For this review, take the finished solid that the model builds, in its own axes (mm). A direction names the side the tool comes from. Round coordinates to 2 decimals unless told otherwise and drop trailing zeros. Order: outer loops, then holes, each group sorted by start corner. A loop starts at its lowest first (then second) coordinate and runs counter-clockwise, first axis right, second up. Notation, with made-up numbers: (84, 74) - (103, 74) arc R17 cw to (103, 78) - close; hole circle Ø1 at (22, 31). An arc over 180 degrees is marked (long way). One line per item, written item: value.
Autodesk Inventor part; units mm, degrees
ref_plane "YZ Plane" through (0, 0, 0) normal (1, 0, 0) x (0, 1, 0)
ref_plane "XZ Plane" through (0, 0, 0) normal (0, 1, 0) x (-1, 0, 0)
ref_plane "XY Plane" through (0, 0, 0) normal (0, 0, 1) x (1, 0, 0)
sketch "Sketch2" plane through (0, 0, 0) normal (0, 1, 0) x (-1, 0, 0)
  line L0 (-9.525, 50.8) -> (9.525, 50.8)
  line L1 (9.525, 50.8) -> (9.525, -50.8)
  line L2 (9.525, -50.8) -> (-9.525, -50.8)
  line L3 (-9.525, -50.8) -> (-9.525, 50.8)
  line L4 (-9.525, 50.8) -> (9.525, -50.8) construction
  line L5 (9.525, 50.8) -> (-9.525, -50.8) construction
  line L6 (-9.525, 50.8) -> (5.715, 50.8)
  line L7 (5.715, 50.8) -> (5.715, 43.18)
  circle A0 centre (5.715, 43.18) radius 2.54
  line L8 (-9.525, -50.8) -> (5.715, -50.8)
  line L9 (5.715, -50.8) -> (5.715, -43.18)
  circle A1 centre (5.715, -43.18) radius 2.54
  point P0 (0, 0)
  dimension "d0" = 19.05
  dimension "d1" = 101.6
  dimension "d2" = 15.24
  dimension "d3" = 7.62
  dimension "d4" = 5.08
  dimension "d10" = 15.24
  dimension "d11" = 7.62
  dimension "d12" = 5.08
extrude "Extrusion3" add sketch "Sketch2" along normal blind 2.54
sketch "Sketch4" plane through (0, 2.54, 0) normal (0, 1, 0) x (1, 0, 0)
  line L0 (9.525, -50.8) -> (9.525, 50.8)
  line L1 (9.525, -50.8) -> (6.985, -50.8)
  line L2 (6.985, -50.8) -> (6.985, 50.8)
  line L3 (6.985, 50.8) -> (9.525, 50.8)
  line L4 (9.525, 50.8) -> (9.525, -50.8)
  point P0 (0, 0)
  dimension "d15" = 2.54
  dimension "d16" = 101.6
extrude "Extrusion4" add sketch "Sketch4" along normal blind 29.21
sketch "Sketch5" plane through (9.525, 0, 50.8) normal (1, 0, 0) x (0, 0, -1)
  line L0 (0, 0) -> (101.6, 0)
  line L1 (101.6, 0) -> (101.6, 31.75)
  line L2 (0, 31.75) -> (101.6, 31.75)
  line L3 (0, 0) -> (0, 31.75)
  line L4 (0, 31.75) -> (101.6, 31.75)
  line L5 (0, 31.75) -> (33.8658, 31.75)
  line L6 (33.8658, 31.75) -> (67.724, 31.75)
  line L7 (16.9329, 31.75) -> (16.9329, 19.05)
  line L8 (50.7949, 31.75) -> (50.7949, 19.05)
  line L9 (67.724, 31.75) -> (101.6, 31.75)
  line L10 (84.662, 31.75) -> (84.662, 19.05)
  line L11 (16.9329, 19.05) -> (4.6829, 19.05)
  line L12 (4.6829, 19.05) -> (29.1829, 19.05)
  line L13 (50.7949, 19.05) -> (38.5449, 19.05)
  line L14 (38.5449, 19.05) -> (63.0449, 19.05)
  circle A0 centre (4.6829, 19.05) radius 1.651
  circle A1 centre (29.1829, 19.05) radius 1.651
  circle A2 centre (38.5449, 19.05) radius 1.651
  circle A3 centre (63.0449, 19.05) radius 1.651
  line L15 (7.4329, 13.55) -> (26.4329, 13.55)
  line L16 (26.4329, 13.55) -> (26.4329, 24.55)
  line L17 (26.4329, 24.55) -> (7.4329, 24.55)
  line L18 (7.4329, 24.55) -> (7.4329, 13.55)
  line L19 (7.4329, 13.55) -> (26.4329, 24.55) construction
  line L20 (26.4329, 13.55) -> (7.4329, 24.55) construction
  line L21 (41.2949, 13.55) -> (60.2949, 13.55)
  line L22 (60.2949, 13.55) -> (60.2949, 24.55)
  line L23 (60.2949, 24.55) -> (41.2949, 24.55)
  line L24 (41.2949, 24.55) -> (41.2949, 13.55)
  line L25 (41.2949, 13.55) -> (60.2949, 24.55) construction
  line L26 (60.2949, 13.55) -> (41.2949, 24.55) construction
  circle A4 centre (84.662, 19.05) radius 3.302
  point P0 (50.8, 0)
  dimension "d19" = 33.8658
  dimension "d20" = 33.8582
  dimension "d21" = 12.7
  dimension "d22" = 12.7
  dimension "d23" = 12.7
  dimension "d24" = 12.25
  dimension "d25" = 24.5
  dimension "d26" = 12.25
  dimension "d27" = 24.5
  dimension "d28" = 3.302
  dimension "d29" = 3.302
  dimension "d30" = 3.302
  dimension "d31" = 3.302
  dimension "d32" = 19
  dimension "d33" = 11
  dimension "d34" = 19
  dimension "d35" = 11
  dimension "d36" = 6.604
extrude "Extrusion5" cut sketch "Sketch5" against normal through all contours A4 | A3 | A2 | L23 L22 L14 L8 | L8 L13 L24 L23 | A0 | L17 L16 L12 L7 | L7 L11 L18 L17 | L12 L16 L15 L18 L11 | L14 L22 L21 L24 L13
properties part number "Pi-Output-Holder"
Item 1: Wall thickness on line 1 (Y direction, x = -3, z = 44); line 2 (X direction, y = 23.5, z = 18) (3 decimals); line 3 (Z direction, x = 8.5, y = 16): over which ranges is each line inside the solid? List them lowest first.
Returned:
line 1: 0 to 2.54
line 2: 6.985 to 9.525
line 3: -50.8 to -35.13, -32.6 to -9.49, 9.51 to 24.37, 43.37 to 50.8
Item 2: Take a section at C-C (z = -43.18). Write out the cut boundary in (x, y) (3 decimals), plus the area to 3 significant figures.
Returned:
outline: (-9.525, 0) - (-8.255, 0) - (-8.255, 2.54) - (-9.525, 2.54) - close; (-3.175, 0) - (9.525, 0) - (9.525, 31.75) - (6.985, 31.75) - (6.985, 2.54) - (-3.175, 2.54) - close
area: 110 mm^2
Item 3: Take a section at A-A (y = 19.05). Write out the cut boundary in (x, z) (3 decimals), plus the area to 3 significant figures.
Returned:
outline: (6.985, -50.8) - (9.525, -50.8) - (9.525, -37.164) - (6.985, -37.164) - close; (6.985, -30.56) - (9.525, -30.56) - (9.525, -13.896) - (6.985, -13.896) - close; (6.985, -10.594) - (9.525, -10.594) - (9.525, -9.495) - (6.985, -9.495) - close; (6.985, 9.505) - (9.525, 9.505) - (9.525, 10.604) - (6.985, 10.604) - close; (6.985, 13.906) - (9.525, 13.906) - (9.525, 24.367) - (6.985, 24.367) - close; (6.985, 43.367) - (9.525, 43.367) - (9.525, 44.466) - (6.985, 44.466) - close; (6.985, 47.768) - (9.525, 47.768) - (9.525, 50.8) - (6.985, 50.8) - close
area: 120 mm^2
Item 4: The part is to be moulded in two halves that separate along Z. For faces 4 (the flat face through (6.985, 10, 1)), 5 (the flat face through (8, 12, 50.8)), 6 (the flat face through (8, 24.55, 0)), 7 (the flat face through (8, 24.55, 34)), say which applies: +Z half, -Z half, draft (parallel to the pull), parting line (faces both ways), or undercut.
Returned:
face 4: draft
face 5: +Z half
face 6: undercut
face 7: undercut
Item 5: Take a section at D-D (z = 22). Write out the cut boundary in (x, y) (3 decimals).
Returned:
outline: (-9.525, 0) - (9.525, 0) - (9.525, 31.75) - (6.985, 31.75) - (6.985, 2.54) - (-9.525, 2.54) - close
Item 6: Take a section at B-B (z = 2.5). Write out the cut boundary in (x, y) (3 decimals).
Returned:
outline: (-9.525, 0) - (9.525, 0) - (9.525, 13.55) - (6.985, 13.55) - (6.985, 2.54) - (-9.525, 2.54) - close; (6.985, 24.55) - (9.525, 24.55) - (9.525, 31.75) - (6.985, 31.75) - close
Item 7: Machinability: for faces 1 (the flat face through (-1, 2.54, 1)), 2 (the flat face through (-9.525, 1, 1)), 3 (the flat face through (8, 19, 43.367)), which of the approach directions +Z, -Z, +X, -X, +Y, -Y give a long, thin tool a straight path to every point of the face, cutting with its end or side? Answer none if there is none.
Returned:
face 1: +Z, -Z, -X, +Y
face 2: +Z, -Z, -X, +Y, -Y
face 3: +X, -X
Item 8: For P1, Ø0.8, axis at x = 7.5, z = -3.5, coming from the -Y side; P2, Ø12, axis at y = 18, z = -20, coming from the -X side (3 decimals), all flat-tipped, find the tip position at first contact; note any pin that passes through.
Returned:
P1: y = 0
P2: x = 6.985
